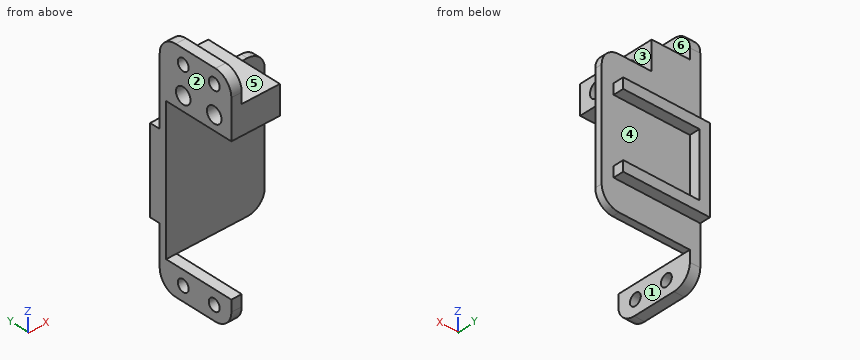
from build123d import *

# Parameters (mm, degrees)
BOSS_EXTRUDE1_DEPTH = 2
SKETCH1_3_W         = 14
SKETCH1_3_H         = 8.25
SKETCH1_3_W_2       = 3
BOSS_EXTRUDE2_DEPTH = 20.4
BOSS_EXTRUDE4_START = -6.075
SKETCH5_W           = 8.05
SKETCH5_H           = 22.4
BOSS_EXTRUDE4_DEPTH = 3
CUT_EXTRUDE1_START  = -6.075
SKETCH2_R           = 1.7
SKETCH2_R_2         = 2.275
CUT_EXTRUDE1_DEPTH  = 54.691836571
FILLET1_R           = 5
SKETCH6_W           = 3
SKETCH6_H           = 18.4
BOSS_EXTRUDE5_DEPTH = 5


with BuildPart() as part:
    # Sketch1 → Boss-Extrude1 (new body)
    with BuildSketch(Plane(origin=(0, 0, 0), x_dir=(1, 0, 0), z_dir=(0, 1, 0))):
        Polygon((22.375, -20.45), (22.375, 20.45), (-3.075, 20.45), (-3.075, 28.7), (-6.075, 28.7), (-6.075, -28.7), (7.925, -28.7), (7.925, -20.45), align=None)
    extrude(amount=BOSS_EXTRUDE1_DEPTH)

    # Sketch1<3> → Boss-Extrude2 (add)
    with BuildSketch(Plane(origin=(0, 0, 0), x_dir=(1, 0, 0), z_dir=(0, 1, 0))):
        with Locations((0.925, -24.575)):
            Rectangle(SKETCH1_3_W, SKETCH1_3_H)
        with Locations((-4.575, 24.575)):
            Rectangle(SKETCH1_3_W_2, SKETCH1_3_H)
    extrude(amount=-BOSS_EXTRUDE2_DEPTH)

    # Sketch5 → Boss-Extrude4 (add)
    with BuildSketch(Plane(origin=(0, 0, 0), x_dir=(0, 0, -1), z_dir=(1, 0, 0)).offset(BOSS_EXTRUDE4_START)):
        with Locations((-32.725, -9.2)):
            Rectangle(SKETCH5_W, SKETCH5_H)
    extrude(amount=BOSS_EXTRUDE4_DEPTH)

    # Sketch2 → Cut-Extrude1 (cut, through all)
    with BuildSketch(Plane(origin=(0, 0, 0), x_dir=(0, 0, -1), z_dir=(1, 0, 0)).offset(CUT_EXTRUDE1_START)):
        with Locations(Location((24.55, -15.05, 0), (0, 0, 180))):
            Circle(SKETCH2_R)
        with Locations(Location((-24.55, -15.05, 0), (0, 0, 180))):
            Circle(SKETCH2_R_2)
        with Locations(Location((-24.55, -5.35, 0), (0, 0, 180))):
            Circle(SKETCH2_R_2)
        with Locations(Location((24.55, -5.35, 0), (0, 0, 180))):
            Circle(SKETCH2_R)
        with Locations(Location((-32.55, -5.35, 0), (0, 0, 180))):
            Circle(SKETCH2_R)
        with Locations(Location((-32.55, -15.05, 0), (0, 0, 180))):
            Circle(SKETCH2_R)
    extrude(amount=CUT_EXTRUDE1_DEPTH, mode=Mode.SUBTRACT)

    # Fillet1
    fillet1_edges = [part.edges().sort_by_distance(p)[0] for p in [
        (22.375, 1, -20.45),
        (22.375, 1, 20.45),
        (-4.575, -20.4, -28.7),
        (-4.575, 2, -28.7),
        (-4.575, 2, 36.75),
        (-4.575, -20.4, 36.75),
    ]]
    fillet(fillet1_edges, radius=FILLET1_R)

    # Sketch6 → Boss-Extrude5 (add)
    with BuildSketch(Plane(origin=(0, 0, 0), x_dir=(1, 0, 0), z_dir=(0, 1, 0))):
        Polygon((-6.075, 12.2), (-6.075, 9.2), (-3.075, 9.2), (18.925, 9.2), (18.925, 12.2), align=None)
        with Locations((-4.575, 0)):
            Rectangle(SKETCH6_W, SKETCH6_H)
        Polygon((-3.075, -9.2), (-6.075, -9.2), (-6.075, -12.2), (18.925, -12.2), (18.925, -9.2), align=None)
    extrude(amount=BOSS_EXTRUDE5_DEPTH)


solid = part.part
Model file for the job. Use its own axes, mm. Face numbers are marked on the shaded views. A direction names the side the tool comes from. Give positions to 0.01 mm unless a question says otherwise; leave off trailing zeros. Order: outer loops, then holes, each group sorted by start corner. A loop starts at its lowest first (then second) coordinate and runs counter-clockwise, first axis right, second up. Notation, with made-up numbers: M 5,78.25 L 23,78.25 A23 cw 23,91.25 Z; hole C 72,82.5 d6. An arc over 180 degrees is marked long. Put each result on its own line as item: value. Start each with the question number.
(1) Drill centre lines: L1, parallel to Z at x = -3.9, y = -5.35 (3 decimals); L2, parallel to Z at x = 1.5, y = -15.05 (3 decimals); L3, parallel to Y at x = 4.5, z = 24.55 (3 decimals). Where is each one in solid material? Low to high. Write a range as [from, to].
(2) Band-saw the part on C-C on x = 0.5. Give the cut face in (y, z) (3 decimals), then the cut area to 3 significant figures.
(3) Pin check, flat tips, straight feed: pin 1 Ø8.5 at (x, z) = (13.5, -8) entering from -Y; pin 2 Ø6.5 at (y, z) = (-7, -26.5) entering from +X (3 decimals); pin 3 Ø9 at (x, y) = (5, -8.5) entering from +Z; pin 4 Ø4 at (y, z) = (-5.35, -24.55) entering from -X (3 decimals). Stop position of each tip, or through.
(4) Tool access for the marked faces 1, 2 and 3: list every direction of +Z, -Z, +X, -X, +Y, -Y with a clear straight run to the whole face (end or side of a thin tool).
(5) Band-saw the part on A-A on z = 24.55. Give the cut face in (x, y) (3 decimals).
(6) Pull direction Z, two halves, no side cores. Call the marked faces 4, 5 and 6: released by +Z, released by -Z, zero draft, split by the parting line, or undercut.
(7) Band-saw the part on D-D on y = -5.35. Give the cut face in (x, z) (3 decimals), then the cut area to 3 significant figures.
(8) Band-saw the part on B-B on y = -9.5. Give the cut face in (x, z) (3 decimals), then the cut area to 3 significant figures.
Results below:
1. L1: z = [-28.7, -26.25], [-22.85, -20.45], [20.45, 22.275], [26.825, 30.85], [34.25, 36.75]
1. L2: z = [20.45, 22.275], [26.825, 28.7]
1. L3: y = [-20.4, -17.325], [-12.775, -7.625], [-3.075, 2]
2. outline: M -20.4,20.45 L 0,20.45 L 0,-20.45 L 2,-20.45 L 2,-12.2 L 5,-12.2 L 5,-9.2 L 2,-9.2 L 2,9.2 L 5,9.2 L 5,12.2 L 2,12.2 L 2,28.7 L -20.4,28.7 Z; hole C -15.05,24.55 d4.55; hole C -5.35,24.55 d4.55
2. area: 252 mm2
3. pin 1: stops at y = 0
3. pin 2: stops at x = -3.075
3. pin 3: stops at z = 28.7
3. pin 4: stops at x = -6.075
4. face 1: -Z, +X, +Y, -Y
4. face 2: +Z, -Z, -X, +Y, -Y
4. face 3: +Z, +X, +Y, -Y
5. outline: M -6.075,-20.4 L 7.925,-20.4 L 7.925,-17.325 L -6.075,-17.325 Z; M -6.075,-12.775 L 7.925,-12.775 L 7.925,-7.625 L -6.075,-7.625 Z; M -6.075,-3.075 L 7.925,-3.075 L 7.925,2 L -6.075,2 Z
6. face 4: undercut
6. face 5: released by +Z
6. face 6: zero draft
7. outline: M -6.075,-28.7 L -3.075,-28.7 L -3.075,-26.25 L -6.075,-26.25 Z; M -6.075,-22.85 L -3.075,-22.85 L -3.075,-20.45 L -6.075,-20.45 Z; M -6.075,20.45 L 7.925,20.45 L 7.925,22.275 L -6.075,22.275 Z; M -6.075,26.825 L 7.925,26.825 L 7.925,28.7 L -3.075,28.7 L -3.075,30.85 L -6.075,30.85 Z; M -6.075,34.25 L -3.075,34.25 L -3.075,36.75 L -6.075,36.75 Z
7. area: 80.3 mm2
8. outline: M -6.075,-28.7 L -3.075,-28.7 L -3.075,-20.45 L -6.075,-20.45 Z; M -6.075,20.45 L 7.925,20.45 L 7.925,28.7 L -3.075,28.7 L -3.075,36.75 L -6.075,36.75 Z
8. area: 164 mm2
